```python
from build123d import *

# Parameters (mm, degrees)
F0_R     = 9.525
F0_W     = 1222.248
F0_H     = 6.35
F1_DEPTH = 6.35
F2_W     = 1222.248
F2_H     = 6.35
F3_DEPTH = 69.85
F4_W     = 65.024
F4_H     = 6.35
F5_DEPTH = 81.026
F6_W     = 65.024
F6_H     = 6.35
F7_DEPTH = 81.026


with BuildPart() as f1:
    # F0 (on Front) → F1 (new body)
    with BuildSketch(Plane.XZ):
        with BuildLine():
            ThreePointArc((-701.675, -33.274), (-699.424995, -36.749995), (-695.510592, -38.1))
            Line((-695.510592, -38.1), (676.275, -38.1))
            ThreePointArc((676.275, -38.1), (680.765128, -36.240128), (682.625, -31.75))
            Line((682.625, -31.75), (682.625, 25.4))
            Line((682.625, 25.4), (611.124, 25.4))
            Line((611.124, 25.4), (611.124, 31.75))
            Line((611.124, 31.75), (-611.124, 31.75))
            Line((-611.124, 31.75), (-611.124, 25.4))
            Line((-611.124, 25.4), (-701.675, 25.4))
            Line((-701.675, 25.4), (-701.675, -33.274))
        make_face()
        with Locations((-663.575, 0)):
            Circle(F0_R, mode=Mode.SUBTRACT)
        with Locations((644.525, 0)):
            Circle(F0_R, mode=Mode.SUBTRACT)
        with Locations((0, 34.925)):
            Rectangle(F0_W, F0_H)
    extrude(amount=F1_DEPTH)

    # F2 (on face) → F3 (join)
    with BuildSketch(Plane.XZ.offset(6.35)):
        with Locations((0, 34.925)):
            Rectangle(F2_W, F2_H)
    extrude(amount=F3_DEPTH)

    # F4 (on face) → F5 (join)
    with BuildSketch(Plane(origin=(-611.124, 0, 0), x_dir=(0, -1, 0), z_dir=(-1, 0, 0))):
        with Locations((43.688, 34.925)):
            Rectangle(F4_W, F4_H)
    extrude(amount=F5_DEPTH)

    # F6 (on face) → F7 (join)
    with BuildSketch(Plane.YZ.offset(611.124)):
        with Locations((-43.688, 34.925)):
            Rectangle(F6_W, F6_H)
    extrude(amount=F7_DEPTH)


solid = f1.part
```
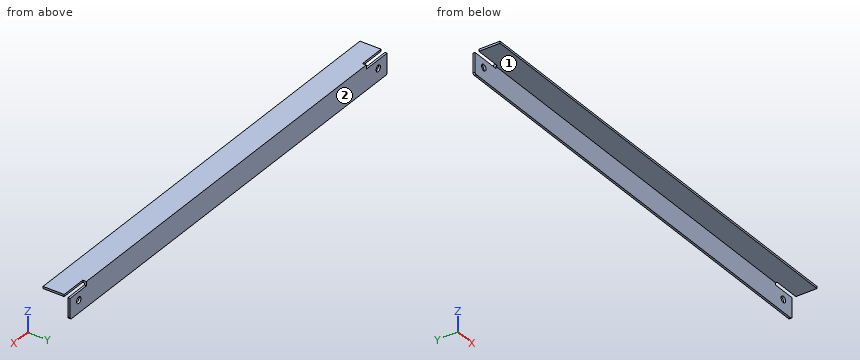
The model under review builds one solid part; all positions refer to its coordinate system, in mm. Face numbers are marked on the shaded views. A direction names the side the tool comes from. Round coordinates to 2 decimals unless told otherwise and drop trailing zeros. Order: outer loops, then holes, each group sorted by start corner. A loop starts at its lowest first (then second) coordinate and runs counter-clockwise, first axis right, second up.
(1) For P1, Ø7, axis at x = -650.5, y = -2.5, coming from the +Z side; P2, Ø2, axis at x = 359.5, y = -38, coming from the -Z side; P3, Ø3.5, axis at y = -6.5, z = 30, coming from the -X side, all flat-tipped, find the tip position at first contact; note any pin that passes through.
Working result:
P1: stops at z = 25.4
P2: stops at z = 31.75
P3: stops at x = -611.12
(2) Wall thickness on L1, parallel to X at y = -4.5, z = -5 (3 decimals); L2, parallel to Z at x = -373, y = -34; L3, parallel to Y at x = -487, z = 26.5: over which ranges is each line inside the solid? List them lowest first.
Working result:
L1: x = -701.675 to -671.682, -655.468 to 636.418, 652.632 to 682.625
L2: z = 31.75 to 38.1
L3: y = -6.35 to 0
(3) Tool access review of the marked faces 1 and 2: name each direction out of +Z, -Z, +X, -X, +Y, -Y from which nothing blocks a thin tool from reaching the whole face with its end or side.
Working result:
face 1: -Z, +X, -X, -Y
face 2: +Z, -Z, +X, -X, +Y
(4) Take a section at B-B, the plane y = -50. State the section outline as (x, z) points, plus the area to 3 significant figures.
Working result:
outline: (-692.15, 31.75) - (692.15, 31.75) - (692.15, 38.1) - (-692.15, 38.1) - close
area: 8,790 mm2
(5) Take a section at A-A, the plane x = -172.5. State the section outline as (y, z) points.
Working result:
outline: (-76.2, 31.75) - (-6.35, 31.75) - (-6.35, -38.1) - (0, -38.1) - (0, 38.1) - (-76.2, 38.1) - close
